```python
from build123d import *

# Parameters (mm, degrees)
SKETCH1_W               = 88.9
SKETCH1_H               = 88.9
BOSS_EXTRUDE1_DEPTH     = 450.85
CUT_EXTRUDE1_DEPTH      = 127
CUT_EXTRUDE2_DEPTH      = 456.211299838
CUT_EXTRUDE2_DEPTH_BACK = 456.211299838
SKETCH3_R               = 12.7


with BuildPart() as part:
    # Sketch1 → Boss-Extrude1 (new body)
    with BuildSketch(Plane(origin=(0, 0, 0), x_dir=(1, 0, 0), z_dir=(0, 1, 0))):
        Rectangle(SKETCH1_W, SKETCH1_H)
    extrude(amount=BOSS_EXTRUDE1_DEPTH)

    # Sketch2 → Cut-Extrude1 (cut)
    with BuildSketch(Plane(origin=(0, 450.85, 0), x_dir=(1, 0, 0), z_dir=(0, 1, 0))):
        with BuildLine():
            Line((-44.45, -44.45), (-1.97e-07, -44.45))
            ThreePointArc((-1.97e-07, -44.45), (-31.430896472, -31.430896376), (-44.45, -6.1e-08))
            Line((-44.45, -6.1e-08), (-44.45, -44.45))
        make_face()
        with BuildLine():
            ThreePointArc((-44.45, -6.1e-08), (-31.430896452, 31.430896396), (-1.8e-08, 44.45))
            Line((-1.8e-08, 44.45), (-44.45, 44.45))
            Line((-44.45, 44.45), (-44.45, -6.1e-08))
        make_face()
        with BuildLine():
            ThreePointArc((-1.8e-08, 44.45), (31.430896417, 31.43089643), (44.45, 0))
            Line((44.45, 0), (44.45, 44.45))
            Line((44.45, 44.45), (-1.8e-08, 44.45))
        make_face()
        with BuildLine():
            Line((44.45, -44.45), (44.45, 0))
            ThreePointArc((44.45, 0), (31.430896354, -31.430896493), (-1.97e-07, -44.45))
            Line((-1.97e-07, -44.45), (44.45, -44.45))
        make_face()
    extrude(amount=-CUT_EXTRUDE1_DEPTH, mode=Mode.SUBTRACT)

    # Sketch3 → Cut-Extrude2 (cut, two sides: drawn at the far end of the back side and taken through both)
    with BuildSketch(Plane.XY.offset(-CUT_EXTRUDE2_DEPTH_BACK)):
        with Locations((0, 273.05)):
            Circle(SKETCH3_R)
    extrude(amount=CUT_EXTRUDE2_DEPTH + CUT_EXTRUDE2_DEPTH_BACK, mode=Mode.SUBTRACT)


solid = part.part
```
Geometry check sheet. Reference: the model listing, model coordinates, mm. A direction names the side the tool comes from. Coordinates: 2 decimals unless noted, no trailing zeros. Loops run counter-clockwise (first coordinate to the right, second up) from the corner with the lowest first, then second, coordinate; pieces in that order, holes last.
Item 1: Sectioned sample at C-C, the plane z = 19. Record the boundary of the cut face in (x, y).
Item 2: Sectioned sample at D-D, the plane x = 23.5. Record the boundary of the cut face in (y, z), then the cut area to 3 significant figures.
Item 3: Sectioned sample at A-A, the plane y = 273.05. Record the boundary of the cut face in (x, z).
Item 4: Thickness scan on line 1 (Y direction, x = 0, z = -10); line 2 (X direction, y = 273.05, z = -21.5); line 3 (X direction, y = 272.5, z = -35.5). Record the ranges inside material, lowest first.
Item 5: Sectioned sample at B-B, the plane x = 6.5. Record the boundary of the cut face in (y, z).
Item 6: Release check for a two-part mould opening along X. For faces 1 (the face through (35, 323.85, 35)), 2 (the face through (6.827, 283.759, -0.622)), 3 (the face through (44.45, 160, 1)) record: released by +X, released by -X, zero draft, split by the parting line, or undercut.
Item 7: Access from +Z, -Z, +X, -X, +Y, -Y to the whole of each face (thin tool, end or side, straight path). Record for faces 4 (the face through (-1, 450.85, -1)), 5 (the face through (-35, 323.85, -34)), 6 (the face through (-35, 323.85, 34)), 7 (the face through (34, 323.85, -35)), 8 (the face through (-1, 160, 44.45)).
Item 8: Go/stop test with flat-tipped pins: pin 1 Ø4 at (y, z) = (375.5, 11) entering from -X; pin 2 Ø20.5 at (x, y) = (0, 273.05) entering from +Z. Record where each tip stops, or that it passes through.
Check result:
1. outline: (-44.45, 0) - (44.45, 0) - (44.45, 323.85) - (40.18, 323.85) - (40.18, 450.85) - (-40.18, 450.85) - (-40.18, 323.85) - (-44.45, 323.85) - close; hole circle Ø25.4 at (0, 273.05)
2. outline: (0, -44.45) - (323.85, -44.45) - (323.85, -37.73) - (450.85, -37.73) - (450.85, 37.73) - (323.85, 37.73) - (323.85, 44.45) - (0, 44.45) - close
2. area: 38,400 mm2
3. outline: (-44.45, -44.45) - (-12.7, -44.45) - (-12.7, 44.45) - (-44.45, 44.45) - close; (12.7, -44.45) - (44.45, -44.45) - (44.45, 44.45) - (12.7, 44.45) - close
4. line 1: y = 0 to 260.35, 285.75 to 450.85
4. line 2: x = -44.45 to -12.7, 12.7 to 44.45
4. line 3: x = -44.45 to -12.69, 12.69 to 44.45
5. outline: (0, -44.45) - (262.14, -44.45) - (262.14, 44.45) - (0, 44.45) - close; (283.96, -44.45) - (323.85, -44.45) - (323.85, -43.97) - (450.85, -43.97) - (450.85, 43.97) - (323.85, 43.97) - (323.85, 44.45) - (283.96, 44.45) - close
6. face 1: zero draft
6. face 2: undercut
6. face 3: released by +X
7. face 4: +Z, -Z, +X, -X, +Y
7. face 5: -Z, -X, +Y
7. face 6: +Z, -X, +Y
7. face 7: -Z, +X, +Y
7. face 8: +Z, +X, -X, +Y, -Y
8. pin 1: stops at x = -43.53
8. pin 2: passes through
